Print and shaded views of the part. All mm, measured from the part's lowest x, y and z. Round coordinates to 2 decimals unless told otherwise and drop trailing zeros. Order: outer loops, then holes, each group sorted by start corner. A loop starts at its lowest first (then second) coordinate and runs counter-clockwise, first axis right, second up. Notation, with made-up numbers: (15.5, -36.5) - (71.5, -36.5) arc R5 ccw to (71.5, -30.5) - close; hole circle Ø4 at (83, -7). An arc over 180 degrees is marked (long way). Return JSON: item names as keys, results as strings. Group by question number.
Item 1: Probe probe 1 along Z at (x, y) = (31.75, 3) (1 decimal); probe 2 along X at (y, z) = (1, 57); probe 3 along Z at (x, y) = (47.5, 5.75). List the from-to ranges inside material, lowest first.
Item 2: Saw through at A-A on z = 12.7. List the corners of the cut face in (x, y) (1 decimal), and give its area (3 significant figures).
Item 3: Saw through at D-D on y = 8.5. State how many separate pieces and enclosed holes the cut face has, and give its area (3 significant figures).
Item 4: Saw through at C-C on z = 50.8. List the corners of the cut face in (x, y) (1 decimal).
Item 5: Saw through at B-B on x = 31.75. List the corners of the cut face in (y, z) (1 decimal), and give its area (3 significant figures).
Item 6: Drop flat-ended pins along their axis: pin 1 (4.5 mm diameter, centred on x = 14.02, z = 33.07, fed in from +Y); pin 2 (1.5 mm diameter, centred on x = 9, y = 3, fed in from +Z). Give the stop position or say it passes through.
Item 7: Two-plate mould, pull along Z, no slides. Class the marked faces 1, 2 and 3: released by +Z, released by -Z, zero draft, split by the parting line, or undercut.
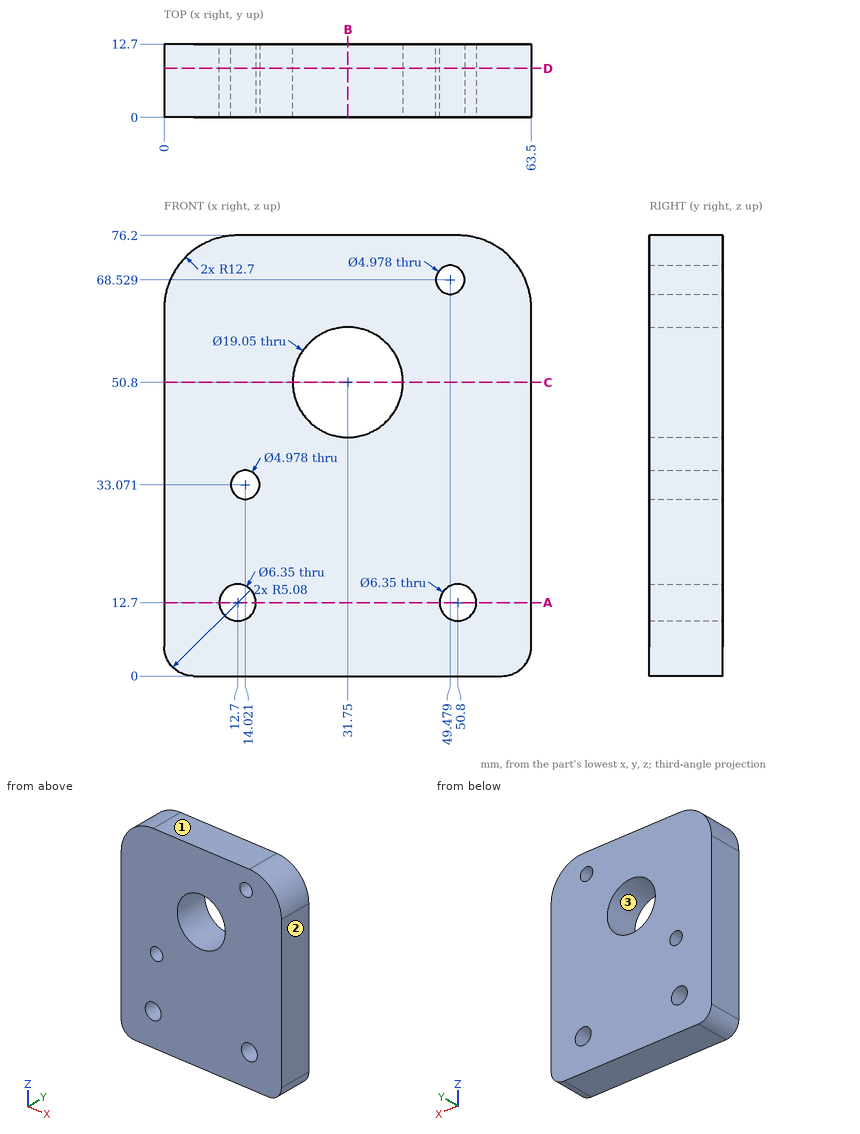
Filled in:
{
 "1": {"probe 1": "z = 0 to 41.3, 60.3 to 76.2", "probe 2": "x = 0 to 24.52, 38.98 to 63.5", "probe 3": "z = 0 to 67.02, 70.04 to 76.2"},
 "2": {"outline": "(0, 0) - (9.5, 0) - (9.5, 12.7) - (0, 12.7) - close; (15.9, 0) - (47.6, 0) - (47.6, 12.7) - (15.9, 12.7) - close; (54, 0) - (63.5, 0) - (63.5, 12.7) - (54, 12.7) - close", "area": "645 mm^2"},
 "3": {"separate pieces": "1", "enclosed holes": "5", "area": "4,370 mm^2"},
 "4": {"outline": "(0, 0) - (22.2, 0) - (22.2, 12.7) - (0, 12.7) - close; (41.3, 0) - (63.5, 0) - (63.5, 12.7) - (41.3, 12.7) - close"},
 "5": {"outline": "(0, 0) - (12.7, 0) - (12.7, 41.3) - (0, 41.3) - close; (0, 60.3) - (12.7, 60.3) - (12.7, 76.2) - (0, 76.2) - close", "area": "726 mm^2"},
 "6": {"pin 1": "passes through", "pin 2": "stops at z = 75.85"},
 "7": {"face 1": "released by +Z", "face 2": "zero draft", "face 3": "undercut"}
}
